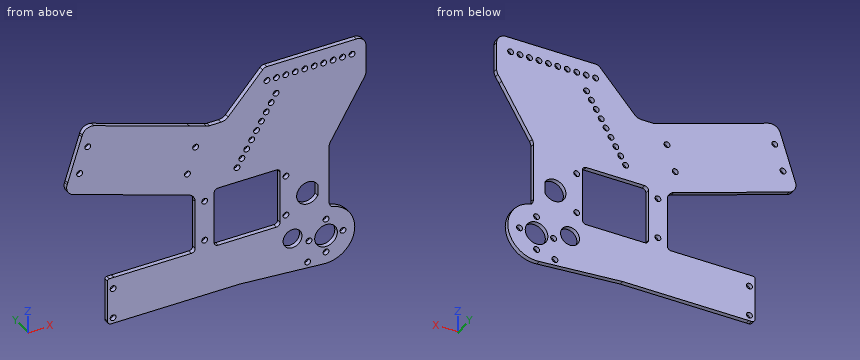
```python
from build123d import *

# Parameters (mm, degrees)
F0_R     = 1.55
F0_R_2   = 5
F0_R_3   = 6
F1_DEPTH = 2.4


with BuildPart() as f1:
    # F0 (on Front) → F1 (new body)
    with BuildSketch(Plane.XZ):
        with BuildLine():
            Line((-108.621812, -36.433733), (-107.21477, -36.41072))
            Line((-107.21477, -36.41072), (-40.668485, -36.41072))
            Line((-40.668485, -36.41072), (3.537217, -39.550132))
            ThreePointArc((3.537217, -39.550132), (20.058172, -26.567412), (7.84607, -9.468945))
            ThreePointArc((7.84607, -9.468945), (7.751121, -9.430233), (7.678601, -9.357742))
            Line((7.678601, -9.357742), (7.442177, -9.002003))
            ThreePointArc((7.442177, -9.002003), (6.8199, -7.679957), (6.606396, -6.234463))
            Line((6.606396, -6.234463), (6.606396, 23.71117))
            ThreePointArc((6.606396, 23.71117), (6.78987, 25.053213), (7.326828, 26.296764))
            Line((7.326828, 26.296764), (23.462316, 53.003568))
            Line((23.462316, 53.003568), (25.392166, 56.197777))
            ThreePointArc((25.392166, 56.197777), (25.929123, 57.441327), (26.112597, 58.78337))
            Line((26.112597, 58.78337), (26.112597, 73.397152))
            ThreePointArc((26.112597, 73.397152), (24.648131, 76.932686), (21.112597, 78.397152))
            Line((21.112597, 78.397152), (-26.302948, 78.397152))
            ThreePointArc((-26.302948, 78.397152), (-27.516081, 78.140928), (-28.521991, 77.416025))
            Line((-28.521991, 77.416025), (-46.817521, 57.3065))
            ThreePointArc((-46.817521, 57.3065), (-48.494039, 56.098327), (-50.515927, 55.671288))
            Line((-50.515927, 55.671288), (-56.604711, 55.671288))
            ThreePointArc((-56.604711, 55.671288), (-57.386884, 55.732846), (-58.149796, 55.916005))
            Line((-58.149796, 55.916005), (-67.178238, 58.849524))
            Line((-67.178238, 58.849524), (-117.661327, 75.252474))
            ThreePointArc((-117.661327, 75.252474), (-121.476365, 74.952224), (-123.961695, 72.042276))
            Line((-123.961695, 72.042276), (-124.270712, 71.09122))
            Line((-124.270712, 71.09122), (-69.03234, 53.143185))
            Line((-69.03234, 53.143185), (-63.194846, 51.246468))
            Line((-63.194846, 51.246468), (-57.696755, 49.46003))
            Line((-57.696755, 49.46003), (-65.13994, 26.552263))
            Line((-65.13994, 26.552263), (-70.638031, 28.338701))
            Line((-70.638031, 28.338701), (-76.448748, 30.317828))
            Line((-76.448748, 30.317828), (-110.062212, 41.239505))
            Line((-110.062212, 41.239505), (-131.687119, 48.265863))
            Line((-131.687119, 48.265863), (-131.996136, 47.314807))
            ThreePointArc((-131.996136, 47.314807), (-131.695887, 43.499769), (-128.785939, 41.014439))
            Line((-128.785939, 41.014439), (-67.669685, 21.156564))
            ThreePointArc((-67.669685, 21.156564), (-65.169685, 19.340208), (-64.21477, 16.401282))
            Line((-64.21477, 16.401282), (-64.21477, -9.363156))
            ThreePointArc((-64.21477, -9.363156), (-64.800556, -10.777369), (-66.21477, -11.363156))
            Line((-66.21477, -11.363156), (-69.222616, -11.363156))
            Line((-69.222616, -11.363156), (-107.21477, -11.363156))
            ThreePointArc((-107.21477, -11.363156), (-107.227913, -11.363199), (-107.241055, -11.363329))
            Line((-107.241055, -11.363329), (-109.66109, -11.379232))
            ThreePointArc((-109.66109, -11.379232), (-110.363945, -11.674431), (-110.654519, -12.379211))
            Line((-110.654519, -12.379211), (-110.654519, -34.434))
            ThreePointArc((-110.654519, -34.434), (-110.057121, -35.859731), (-108.621812, -36.433733))
        make_face()
        with Locations((-107.654519, -33.41072)):
            Circle(F0_R, mode=Mode.SUBTRACT)
        with Locations((-107.654519, -17.41072)):
            Circle(F0_R, mode=Mode.SUBTRACT)
        with Locations((-59.21477, -6.363156)):
            Circle(F0_R, mode=Mode.SUBTRACT)
        with Locations((-59.21477, 15.033994)):
            Circle(F0_R, mode=Mode.SUBTRACT)
        with Locations((-4.71477, -35.80329)):
            Circle(F0_R, mode=Mode.SUBTRACT)
        with Locations((5.001765, -33.41072)):
            Circle(F0_R, mode=Mode.SUBTRACT)
        with Locations((-3.998235, -24.41072)):
            Circle(F0_R, mode=Mode.SUBTRACT)
        with Locations((-12.71477, -20.41072)):
            Circle(F0_R_2, mode=Mode.SUBTRACT)
        with Locations((5.001765, -24.41072)):
            Circle(F0_R_3, mode=Mode.SUBTRACT)
        with Locations((5.001765, -15.41072)):
            Circle(F0_R, mode=Mode.SUBTRACT)
        with Locations((14.001765, -24.41072)):
            Circle(F0_R, mode=Mode.SUBTRACT)
        with BuildLine():
            Line((-21.21477, -11.363156), (-52.21477, -11.363156))
            ThreePointArc((-52.21477, -11.363156), (-53.628983, -10.777369), (-54.21477, -9.363156))
            Line((-54.21477, -9.363156), (-54.21477, 18.033994))
            ThreePointArc((-54.21477, 18.033994), (-53.628983, 19.448208), (-52.21477, 20.033994))
            Line((-52.21477, 20.033994), (-21.21477, 20.033994))
            ThreePointArc((-21.21477, 20.033994), (-19.800556, 19.448208), (-19.21477, 18.033994))
            Line((-19.21477, 18.033994), (-19.21477, -9.363156))
            ThreePointArc((-19.21477, -9.363156), (-19.800556, -10.777369), (-21.21477, -11.363156))
        make_face(mode=Mode.SUBTRACT)
        with Locations((-16.21477, -6.363156)):
            Circle(F0_R, mode=Mode.SUBTRACT)
        with Locations((-16.21477, 15.033994)):
            Circle(F0_R, mode=Mode.SUBTRACT)
        with BuildLine():
            ThreePointArc((0.650781, -0.909588), (-10.547568, 2.086604), (0.650781, 5.082797))
            Line((0.650781, 5.082797), (0.650781, -0.909588))
        make_face(mode=Mode.SUBTRACT)
        with Locations((-42.103694, 27.951924)):
            Circle(F0_R, mode=Mode.SUBTRACT)
        with Locations((-39.518101, 32.231493)):
            Circle(F0_R, mode=Mode.SUBTRACT)
        with Locations((-36.932508, 36.511062)):
            Circle(F0_R, mode=Mode.SUBTRACT)
        with Locations((-34.346915, 40.79063)):
            Circle(F0_R, mode=Mode.SUBTRACT)
        with Locations((-31.761322, 45.070199)):
            Circle(F0_R, mode=Mode.SUBTRACT)
        with Locations((-29.175728, 49.349768)):
            Circle(F0_R, mode=Mode.SUBTRACT)
        with Locations((-26.590135, 53.629336)):
            Circle(F0_R, mode=Mode.SUBTRACT)
        with Locations((-24.004542, 57.908905)):
            Circle(F0_R, mode=Mode.SUBTRACT)
        with Locations((-21.418949, 62.188474)):
            Circle(F0_R, mode=Mode.SUBTRACT)
        with Locations((-26.247763, 70.747611)):
            Circle(F0_R, mode=Mode.SUBTRACT)
        with Locations((-21.247763, 70.747611)):
            Circle(F0_R, mode=Mode.SUBTRACT)
        with Locations((-16.247763, 70.747611)):
            Circle(F0_R, mode=Mode.SUBTRACT)
        with Locations((-11.247763, 70.747611)):
            Circle(F0_R, mode=Mode.SUBTRACT)
        with Locations((-6.247763, 70.747611)):
            Circle(F0_R, mode=Mode.SUBTRACT)
        with Locations((-1.247763, 70.747611)):
            Circle(F0_R, mode=Mode.SUBTRACT)
        with Locations((3.752237, 70.747611)):
            Circle(F0_R, mode=Mode.SUBTRACT)
        with Locations((8.752237, 70.747611)):
            Circle(F0_R, mode=Mode.SUBTRACT)
        with Locations((13.752237, 70.747611)):
            Circle(F0_R, mode=Mode.SUBTRACT)
        with Locations((18.752237, 70.747611)):
            Circle(F0_R, mode=Mode.SUBTRACT)
        Polygon((-124.270712, 71.09122), (-131.687119, 48.265863), (-110.062212, 41.239505), (-76.448748, 30.317828), (-70.638031, 28.338701), (-65.13994, 26.552263), (-57.696755, 49.46003), (-63.194846, 51.246468), (-69.03234, 53.143185), align=None)
        with Locations((-68.350138, 32.85263)):
            Circle(F0_R, mode=Mode.SUBTRACT)
        with Locations((-63.997123, 46.249832)):
            Circle(F0_R, mode=Mode.SUBTRACT)
        with Locations((-125.386752, 51.476061)):
            Circle(F0_R, mode=Mode.SUBTRACT)
        with Locations((-121.060514, 64.790852)):
            Circle(F0_R, mode=Mode.SUBTRACT)
    extrude(amount=F1_DEPTH)


solid = f1.part
```
The model under review builds one solid part; all positions refer to its coordinate system, in mm. Give positions to 0.01 mm unless a question says otherwise; leave off trailing zeros. Loops run counter-clockwise (first coordinate to the right, second up) from the corner with the lowest first, then second, coordinate; pieces in that order, holes last. Notation, with made-up numbers: (31, 76.25) - (42, 76.25) arc R17 ccw to (42, 88.25) - close; hole circle Ø9 at (28.25, 71.5). An arc over 180 degrees is marked (long way). Answer as a JSON object with one key per item and string values.
Q1. Add section A-A on x = -75. State the section outline as (y, z) points.
Worked out:
{"outline": "(-2.4, -36.41) - (0, -36.41) - (0, -11.36) - (-2.4, -11.36) - close; (-2.4, 23.54) - (0, 23.54) - (0, 61.39) - (-2.4, 61.39) - close"}
Q2. Insertion check: pin 1 (3 mm diameter, centred on x = -31.76, z = 45.07, fed in from -Y); pin 2 (0.7 mm diameter, centred on y = -1.5, z = 1, fed in from -X); pin 3 (1 mm diameter, centred on y = -2, z = -26, fed in from -X). Each pin has a flat end and moves straight along its axis. Give the tip position at first contact, or say it passes through.
Worked out:
{"pin 1": "passes through", "pin 2": "stops at x = -64.21", "pin 3": "stops at x = -110.65"}
Q3. Add section B-B on y = -1.15. Count the separate pieces of the cut face and the enclosed holes in it, plus the area to 3 significant figures.
Worked out:
{"separate pieces": "1", "enclosed holes": "38", "area": "10,600 mm^2"}
Q4. To check wall thickness, follow line 1 along Z through (x, y) = (-59, -0.15); line 2 along Z through (x, y) = (-49, -1.6); line 3 along X through (y, z) = (-2.2, -34.5). State the ranges of each line that lie inside material, in increasing order.
Worked out:
{"line 1": "z = -36.41 to -7.9, -4.83 to 13.5, 16.57 to 56.19", "line 2": "z = -36.41 to -11.36, 20.03 to 55.91", "line 3": "x = -110.65 to -108.76, -106.55 to -5.55, -3.88 to 3.9, 6.1 to 16.38"}
